For this review, take the finished solid that the model builds, in its own axes (mm). Round coordinates to 2 decimals unless told otherwise and drop trailing zeros. Order: outer loops, then holes, each group sorted by start corner. A loop starts at its lowest first (then second) coordinate and runs counter-clockwise, first axis right, second up. Notation, with made-up numbers: M -28.5,13.25 L -4.5,13.25 A28 cw -4.5,31.25 Z; hole C -37,-16.75 d10. An arc over 180 degrees is marked long. Use a Markdown table: item, result.
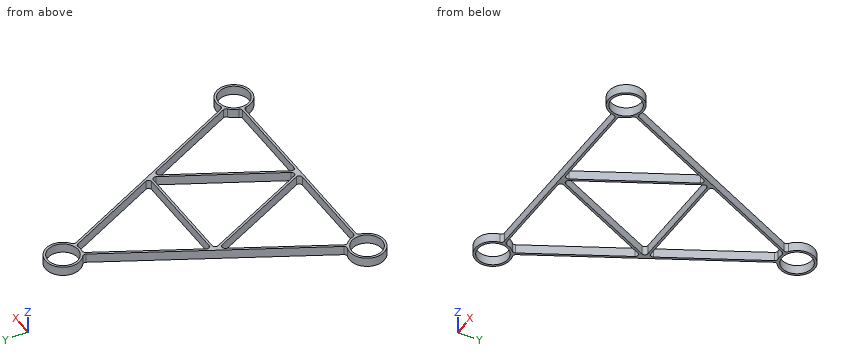
from build123d import *

# Parameters (mm, degrees)
F0_R     = 9.9
F1_DEPTH = 6
F2_R     = 2


with BuildPart() as f1:
    # F0 (on Top) → F1 (new body)
    with BuildSketch(Plane.XY):
        with BuildLine():
            Line((-66.35, -77.75), (66.35, -77.75))
            ThreePointArc((66.35, -77.75), (87.447419, -83.743335), (72.651765, -67.55353))
            Line((72.651765, -67.55353), (5.098235, 67.55353))
            ThreePointArc((5.098235, 67.55353), (0, 89.15), (-5.098235, 67.55353))
            Line((-5.098235, 67.55353), (-72.651765, -67.55353))
            ThreePointArc((-72.651765, -67.55353), (-87.447419, -83.743335), (-66.35, -77.75))
        make_face()
        with Locations((-77.75, -77.75)):
            Circle(F0_R, mode=Mode.SUBTRACT)
        with BuildLine():
            Line((-1.674783, -76.25), (-66.449115, -76.25))
            ThreePointArc((-66.449115, -76.25), (-68.052581, -71.756665), (-71.35445, -68.313002))
            Line((-71.35445, -68.313002), (-38.373599, -2.351301))
            Line((-38.373599, -2.351301), (-1.674783, -76.25))
        make_face(mode=Mode.SUBTRACT)
        with Locations((77.75, -77.75)):
            Circle(F0_R, mode=Mode.SUBTRACT)
        Polygon((37.533359, -0.67082), (0, -76.25), (-37.533359, -0.67082), align=None, mode=Mode.SUBTRACT)
        with BuildLine():
            Line((38.373599, -2.351301), (71.35445, -68.313002))
            ThreePointArc((71.35445, -68.313002), (68.052581, -71.756665), (66.449115, -76.25))
            Line((66.449115, -76.25), (1.674783, -76.25))
            Line((1.674783, -76.25), (38.373599, -2.351301))
        make_face(mode=Mode.SUBTRACT)
        with Locations((0, 77.75)):
            Circle(F0_R, mode=Mode.SUBTRACT)
        with BuildLine():
            ThreePointArc((-3.712269, 66.971361), (0, 66.35), (3.712269, 66.971361))
            Line((3.712269, 66.971361), (36.783359, 0.82918))
            Line((36.783359, 0.82918), (-36.783359, 0.82918))
            Line((-36.783359, 0.82918), (-3.712269, 66.971361))
        make_face(mode=Mode.SUBTRACT)
    extrude(amount=F1_DEPTH)

    # F2
    f2_edges = [f1.edges().sort_by_distance(p)[0] for p in [
        (-37.533359, -0.67082, 3),
        (-3.712269, 66.971361, 3),
        (5.098235, 67.55353, 3),
        (3.712269, 66.971361, 3),
        (-5.098235, 67.55353, 3),
        (38.373599, -2.351301, 3),
        (37.533359, -0.67082, 3),
        (36.783359, 0.82918, 3),
        (1.674783, -76.25, 3),
        (0, -76.25, 3),
        (-1.674783, -76.25, 3),
        (71.35445, -68.313002, 3),
        (66.449115, -76.25, 3),
        (66.35, -77.75, 3),
        (72.651765, -67.55353, 3),
        (-66.35, -77.75, 3),
        (-72.651765, -67.55353, 3),
        (-66.449115, -76.25, 3),
        (-71.35445, -68.313002, 3),
        (-36.783359, 0.82918, 3),
        (-38.373599, -2.351301, 3),
    ]]
    fillet(f2_edges, radius=F2_R)


solid = f1.part
Q1. Add section D-D (z = 4). Give the number of separate pieces and of enclosed holes in the cut face, then the cut area to 3 significant figures.
Determined:
| item | result |
|---|---|
| separate pieces | 1 |
| enclosed holes | 7 |
| area | 1,350 mm^2 |
Q2. Wall thickness on line 1 along Y through (x, z) = (69, 4); line 2 along X through (y, z) = (-34.5, 5.05) (3 decimals); line 3 along Y through (x, z) = (-36, 3.6): over which ranges is each line inside the solid? List them lowest first. Write a range as [from, to].
Determined:
| item | result |
|---|---|
| line 1 | y = [-85.06, -82.38], [-73.12, -70.44], [-63.6, -60.25] |
| line 2 | x = [-56.125, -54.448], [-22.408, -20.733], [20.733, 22.408], [54.448, 56.125] |
| line 3 | y = [-77.75, -76.25], [-7.13, -3.76], [-1.61, 5.75] |
Q3. Add section C-C (y = -33). Write out the cut boundary in (x, z) (3 decimals), then the cut area to 3 significant figures.
Determined:
| item | result |
|---|---|
| outline | M -55.375,0 L -53.698,0 L -53.698,6 L -55.375,6 Z; M -23.153,0 L -21.478,0 L -21.478,6 L -23.153,6 Z; M 21.478,0 L 23.153,0 L 23.153,6 L 21.478,6 Z; M 53.698,0 L 55.375,0 L 55.375,6 L 53.698,6 Z |
| area | 40.2 mm^2 |
Q4. Add section A-A (y = 77.75). Write out the cut boundary in (x, z).
Determined:
| item | result |
|---|---|
| outline | M -11.4,0 L -9.9,0 L -9.9,6 L -11.4,6 Z; M 9.9,0 L 11.4,0 L 11.4,6 L 9.9,6 Z |
Q5. Add section B-B (x = 77.75). Write out the cut boundary in (y, z).
Determined:
| item | result |
|---|---|
| outline | M -89.15,0 L -87.65,0 L -87.65,6 L -89.15,6 Z; M -67.85,0 L -66.35,0 L -66.35,6 L -67.85,6 Z |
Q6. Clearance check with flat-ended pins moving along their axes: pin 1 (3 mm diameter, centred on x = -16.5, z = 4, fed in from +Y); pin 2 (1 mm diameter, centred on y = -54.5, z = 3, fed in from +X) (3 decimals); pin 3 (1 mm diameter, centred on y = -7, z = 5, fed in from +X) (3 decimals). State where each tip first meets the part, or that it passes through.
Determined:
| item | result |
|---|---|
| pin 1 | stops at y = 47.75 |
| pin 2 | stops at x = 66.375 |
| pin 3 | stops at x = 42.625 |
